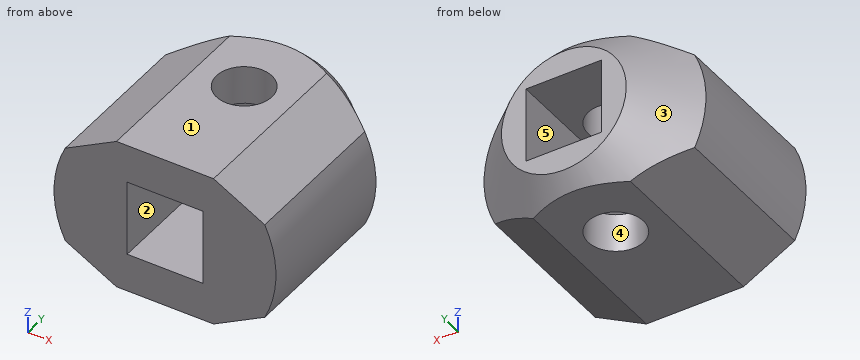
from build123d import *

# Parameters (mm, degrees)
CUT_EXTRUDE4_DEPTH      = 38.150064549
CUT_EXTRUDE5_DEPTH      = 36.286361331
CUT_EXTRUDE5_DEPTH_BACK = 36.286361331
SKETCH3_R               = 4
SKETCH4_W               = 10.922
SKETCH4_H               = 10.922
CUT_EXTRUDE6_DEPTH      = 36.286361446


with BuildPart() as part:
    # Sketch1 → Revolve1 (revolve)
    with BuildSketch(Plane.XY, mode=Mode.PRIVATE) as revolve1_sk:
        Polygon((9, 29.464), (16, 22.464), (16, 0), (4.925, 0), (4.925, 29.464), align=None)
    revolve(revolve1_sk.sketch.rotate(Axis((0, 0, 0), (0, 1, 0)), 90), axis=Axis((0, 0, 0), (0, 1, 0)))

    # Sketch2 → Cut-Extrude4 (cut, through all)
    with BuildSketch(Plane(origin=(0, 0, 0), x_dir=(1, 0, 0), z_dir=(0, 1, 0))):
        with BuildLine():
            Line((7, 11), (14.38749457, 7))
            ThreePointArc((14.38749457, 7), (0, 16), (-14.38749457, 7))
            Line((-14.38749457, 7), (-7, 11))
            Line((-7, 11), (7, 11))
        make_face()
        with BuildLine():
            ThreePointArc((14.38749457, -7), (0, -16), (-14.38749457, -7))
            Line((-14.38749457, -7), (-7, -11))
            Line((-7, -11), (7, -11))
            Line((7, -11), (14.38749457, -7))
        make_face()
    extrude(amount=CUT_EXTRUDE4_DEPTH, mode=Mode.SUBTRACT)

    # Sketch3 → Cut-Extrude5 (cut, two sides: drawn at the far end of the back side and taken through both)
    with BuildSketch(Plane.XY.offset(-CUT_EXTRUDE5_DEPTH_BACK)):
        with Locations((0, 17.78)):
            Circle(SKETCH3_R)
    extrude(amount=CUT_EXTRUDE5_DEPTH + CUT_EXTRUDE5_DEPTH_BACK, mode=Mode.SUBTRACT)

    # Sketch4 → Cut-Extrude6 (cut, through all)
    with BuildSketch(Plane.XZ):
        Rectangle(SKETCH4_W, SKETCH4_H)
    extrude(amount=-CUT_EXTRUDE6_DEPTH, mode=Mode.SUBTRACT)


solid = part.part
Design review of the part built by this model. Coordinates are the model's own, in mm. Face numbers are marked on the shaded views. A direction names the side the tool comes from. Coordinates: 2 decimals unless noted, no trailing zeros. Order: outer loops, then holes, each group sorted by start corner. A loop starts at its lowest first (then second) coordinate and runs counter-clockwise, first axis right, second up. Notation, with made-up numbers: (63, 21.25) - (105, 21.25) arc R18 ccw to (105, 25.25) - close; hole circle Ø5 at (22, 42.5). An arc over 180 degrees is marked (long way). Put each result on its own line as item: value.
1) Take a section at A-A, the plane y = 2.25. Give the boundary of the cut face in (x, z).
Response values:
outline: (-14.39, -7) - (-7, -11) - (7, -11) - (14.39, -7) arc R16 ccw to (14.39, 7) - (7, 11) - (-7, 11) - (-14.39, 7) arc R16 ccw to start; hole (-5.46, -5.46) - (5.46, -5.46) - (5.46, 5.46) - (-5.46, 5.46) - close
2) Wall thickness on L1, parallel to Z at x = 4.5, y = 4.25; L2, parallel to Y at x = 0, z = 6.95; L3, parallel to X at y = 12, z = -0.25: over which ranges is each line inside the solid? List them lowest first. Write a range as from..to.
Response values:
L1: z = -11..-5.46, 5.46..11
L2: y = 0..13.78, 21.78..29.46
L3: x = -16..-5.46, 5.46..16
3) Take a section at B-B, the plane z = 0. Give the boundary of the cut face in (x, y).
Response values:
outline: (-16, 0) - (-5.46, 0) - (-5.46, 29.46) - (-9, 29.46) - (-16, 22.46) - close; (5.46, 0) - (16, 0) - (16, 22.46) - (9, 29.46) - (5.46, 29.46) - close
4) Tool access review of the marked faces 4 and 5: name each direction out of +Z, -Z, +X, -X, +Y, -Y from which nothing blocks a thin tool from reaching the whole face with its end or side.
Response values:
face 4: +Z, -Z
face 5: +Y, -Y
5) The part is to be moulded in two halves that separate along Z. For the marked faces 1, 2 and 3, say which applies: released by +Z, released by -Z, zero draft, split by the parting line, or undercut.
Response values:
face 1: released by +Z
face 2: undercut
face 3: split by the parting line
6) Take a section at D-D, the plane y = 17.78. Give the boundary of the cut face in (x, z).
Response values:
outline: (-14.39, -7) - (-7, -11) - (-4, -11) - (-4, -5.46) - (-5.46, -5.46) - (-5.46, 5.46) - (-4, 5.46) - (-4, 11) - (-7, 11) - (-14.39, 7) arc R16 ccw to start; (4, -11) - (7, -11) - (14.39, -7) arc R16 ccw to (14.39, 7) - (7, 11) - (4, 11) - (4, 5.46) - (5.46, 5.46) - (5.46, -5.46) - (4, -5.46) - close
7) Take a section at C-C, the plane x = 0. Give the boundary of the cut face in (y, z).
Response values:
outline: (0, -11) - (13.78, -11) - (13.78, -5.46) - (0, -5.46) - close; (0, 5.46) - (13.78, 5.46) - (13.78, 11) - (0, 11) - close; (21.78, -11) - (27.46, -11) - (29.46, -9) - (29.46, -5.46) - (21.78, -5.46) - close; (21.78, 5.46) - (29.46, 5.46) - (29.46, 9) - (27.46, 11) - (21.78, 11) - close
8) Insertion check: P1, Ø2, axis at y = 24, z = 6, coming from the -X side; P2, Ø8, axis at y = 6, z = 5.5, coming from the -X side; P3, Ø5, axis at y = 8, z = -8, coming from the +X side (3 decimals). Each pin has a flat end and moves straight along its axis. Give the tip position at first contact, or say it passes through.
Response values:
P1: stops at x = -14.33
P2: stops at x = -15.93
P3: stops at x = 15.025
